Geometry: final body of the model. Coordinates: model frame, mm. Face numbers are marked on the shaded views. A direction names the side the tool comes from. Coordinates: 2 decimals unless noted, no trailing zeros. Order: outer loops, then holes, each group sorted by start corner. A loop starts at its lowest first (then second) coordinate and runs counter-clockwise, first axis right, second up. Notation, with made-up numbers: (77, -27) -> (119, -27) arc R20 cw to (119, -14) -> close; hole circle Ø9 at (2, 42). An arc over 180 degrees is marked (long way). Answer in a Markdown table with one row per item. Add a question column.
1) Pull-direction query (Z, two-part tool) for the marked faces 3, 4 and 5; classes: +Z half, -Z half, draft (parallel to the pull), parting line (faces both ways), or undercut.
2) Set-up query: the marked faces 1 and 2. Return all of +Z, -Z, +X, -X, +Y, -Y with unobstructed straight access to the full face (end or side cutting, diameter ignored); none if empty.
3) Section query D-D on z = 7.75. Return the cut outline in (x, y) (3 decimals).
4) Contact query for flat-ended pins moving along their axis: P1, Ø3.5, axis at y = 6.91, z = 6.91, coming from the +X side (3 decimals); P2, Ø5.5, axis at y = -1, z = 0.5, coming from the +X side; P3, Ø1.5, axis at x = 3.5, y = 9, coming from the -Z side. Output: stop coordinate, or through.
5) Section query A-A on y = 0. Return the cut outline in (x, z) (3 decimals), then the cut area to 3 significant figures.
6) Ray query, line 1 (Y direction, x = 3.15, z = 0); line 2 (Y direction, x = 3.9, z = -6.75); line 3 (Z direction, x = 0.75, y = -6.5). Return the intervals inside material, ascending. Write a range as from..to.
7) Section query C-C on x = 3.35. Count the separate pieces of the cut face and the enclosed holes in it, then the cut area to 3 significant figures.
```python
from build123d import *

# Parameters (mm, degrees)
SKETCH1_R           = 12.7
SKETCH1_R_2         = 1.35255
BOSS_EXTRUDE1_DEPTH = 4.445
SKETCH2_R           = 6.35
CUT_EXTRUDE1_DEPTH  = 0.762
SKETCH3_R           = 3.302
CUT_EXTRUDE2_DEPTH  = 1.778
SKETCH4_R           = 1.8288
CUT_EXTRUDE3_DEPTH  = 2.905


with BuildPart() as part:
    # Sketch1 → Boss-Extrude1 (new body)
    with BuildSketch(Plane(origin=(0, 0, 0), x_dir=(0, 0, -1), z_dir=(1, 0, 0))):
        Circle(SKETCH1_R)
        with Locations((0, 9.779)):
            Circle(SKETCH1_R_2, mode=Mode.SUBTRACT)
        with Locations((6.914797213, 6.914797213)):
            Circle(SKETCH1_R_2, mode=Mode.SUBTRACT)
        with Locations((9.779, 0)):
            Circle(SKETCH1_R_2, mode=Mode.SUBTRACT)
        with Locations((6.914797213, -6.914797213)):
            Circle(SKETCH1_R_2, mode=Mode.SUBTRACT)
        with Locations((0, -9.779)):
            Circle(SKETCH1_R_2, mode=Mode.SUBTRACT)
        with Locations((-6.914797213, -6.914797213)):
            Circle(SKETCH1_R_2, mode=Mode.SUBTRACT)
        with Locations((-9.779, 0)):
            Circle(SKETCH1_R_2, mode=Mode.SUBTRACT)
        with Locations((-6.914797213, 6.914797213)):
            Circle(SKETCH1_R_2, mode=Mode.SUBTRACT)
    extrude(amount=BOSS_EXTRUDE1_DEPTH)

    # Sketch2 → Cut-Extrude1 (cut)
    with BuildSketch(Plane(origin=(4.445, 0, 0), x_dir=(0, 0, -1), z_dir=(1, 0, 0))):
        Circle(SKETCH2_R)
    extrude(amount=-CUT_EXTRUDE1_DEPTH, mode=Mode.SUBTRACT)

    # Sketch3 → Cut-Extrude2 (cut)
    with BuildSketch(Plane(origin=(3.683, 0, 0), x_dir=(0, 0, -1), z_dir=(1, 0, 0))):
        Circle(SKETCH3_R)
    extrude(amount=-CUT_EXTRUDE2_DEPTH, mode=Mode.SUBTRACT)

    # Sketch4 → Cut-Extrude3 (cut, through all)
    with BuildSketch(Plane(origin=(1.905, 0, 0), x_dir=(0, 0, -1), z_dir=(1, 0, 0))):
        Circle(SKETCH4_R)
    extrude(amount=-CUT_EXTRUDE3_DEPTH, mode=Mode.SUBTRACT)


solid = part.part
```
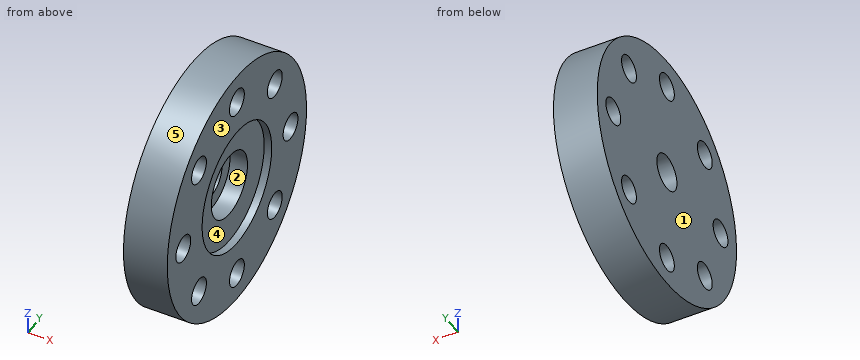
Result:
| question | item | result |
|---|---|---|
| 1 | face 3 | draft |
| 1 | face 4 | undercut |
| 1 | face 5 | parting line |
| 2 | face 1 | +Z, -Z, -X, +Y, -Y |
| 2 | face 2 | +X |
| 3 | outline | (0, -10.061) -> (4.445, -10.061) -> (4.445, -7.979) -> (0, -7.979) -> close; (0, -5.851) -> (4.445, -5.851) -> (4.445, 5.851) -> (0, 5.851) -> close; (0, 7.979) -> (4.445, 7.979) -> (4.445, 10.061) -> (0, 10.061) -> close |
| 4 | P1 | x = 4.445 |
| 4 | P2 | x = 3.68 |
| 4 | P3 | z = -9.66 |
| 5 | outline | (0, -12.7) -> (4.445, -12.7) -> (4.445, -11.132) -> (0, -11.132) -> close; (0, -8.426) -> (4.445, -8.426) -> (4.445, -6.35) -> (3.683, -6.35) -> (3.683, -3.302) -> (1.905, -3.302) -> (1.905, -1.829) -> (0, -1.829) -> close; (0, 1.829) -> (1.905, 1.829) -> (1.905, 3.302) -> (3.683, 3.302) -> (3.683, 6.35) -> (4.445, 6.35) -> (4.445, 8.426) -> (0, 8.426) -> close; (0, 11.132) -> (4.445, 11.132) -> (4.445, 12.7) -> (0, 12.7) -> close |
| 5 | area | 60.5 mm2 |
| 6 | line 1 | -12.7..-11.13, -8.43..-3.3, 3.3..8.43, 11.13..12.7 |
| 6 | line 2 | -10.76..-8.26, -5.57..5.57, 8.26..10.76 |
| 6 | line 3 | -10.91..-8.2, -5.63..5.63, 8.2..10.91 |
| 7 | separate pieces | 1 |
| 7 | enclosed holes | 9 |
| 7 | area | 426 mm2 |
